```python
from build123d import *

# Parameters (mm, degrees)
SKETCH_1_W            = 179.605
SKETCH_1_H            = 31
EXTRUDE_1_DEPTH       = 8
HOLE_WIZARD_1_4_201_D = 5.1054
HOLE_WIZARD_3_8_161_D = 7.9375
FILLET_1_R            = 4


with BuildPart() as part:
    # Эскиз1 → Бобышка-Вытянуть1 (new body)
    with BuildSketch(Plane(origin=(0, 0, 0), x_dir=(1, 0, 0), z_dir=(0, 1, 0))):
        with Locations((89.8025, 15.5)):
            Rectangle(SKETCH_1_W, SKETCH_1_H)
    extrude(amount=EXTRUDE_1_DEPTH)

    # Отверстие обработанное метчиком 1/4-201 (through all)
    with Locations(Plane(origin=(0, 0, 0), x_dir=(-1, 0, 0), z_dir=(0, -1, 0))):
        with Locations((-10.475, 25), (-18.825, 25), (-27.175, 25), (-35.525, 25), (-43.875, 25), (-52.225, 25), (-60.575, 25), (-68.925, 25), (-77.275, 25), (-85.625, 25), (-93.975, 25), (-102.325, 25), (-110.675, 25), (-119.025, 25), (-127.375, 25), (-135.725, 25), (-144.075, 25), (-152.425, 25), (-160.775, 25), (-169.125, 25), (-169.125, 6), (-160.775, 6), (-152.425, 6), (-144.075, 6), (-135.725, 6), (-127.375, 6), (-119.025, 6), (-110.675, 6), (-102.325, 6), (-93.975, 6), (-85.625, 6), (-77.275, 6), (-68.925, 6), (-60.575, 6), (-52.225, 6), (-43.875, 6), (-35.525, 6), (-27.175, 6), (-18.825, 6), (-10.475, 6)):
            Hole(HOLE_WIZARD_1_4_201_D / 2)

    # Отверстие обработанное метчиком 3/8-161 (through all)
    with Locations(Plane(origin=(0, 0, 0), x_dir=(-1, 0, 0), z_dir=(0, -1, 0))):
        with Locations((-9.095, 15.5), (-20.62, 15.5), (-32.15, 15.5), (-43.68, 15.5), (-55.21, 15.5), (-66.74, 15.5), (-78.27, 15.5), (-89.8, 15.5), (-101.33, 15.5), (-112.86, 15.5), (-124.39, 15.5), (-135.92, 15.5), (-147.45, 15.5), (-158.98, 15.5), (-170.51, 15.5)):
            Hole(HOLE_WIZARD_3_8_161_D / 2)

    # Скругление1
    fillet_1_edges = [part.edges().sort_by_distance(p)[0] for p in [
        (0, 4, 0),
        (0, 4, -31),
        (179.605, 4, -31),
        (179.605, 4, 0),
    ]]
    fillet(fillet_1_edges, radius=FILLET_1_R)


solid = part.part
```
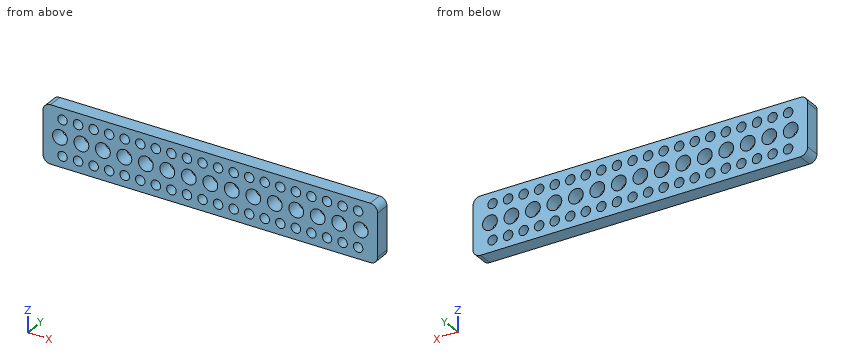
Check sheet for the modelled part. Datum: model origin and axes. Units: mm. Give positions to 0.01 mm unless a question says otherwise; leave off trailing zeros. Order: outer loops, then holes, each group sorted by start corner. A loop starts at its lowest first (then second) coordinate and runs counter-clockwise, first axis right, second up. Notation, with made-up numbers: (27, -16.5) -> (77, -16.5) arc R18 ccw to (77, 2.5) -> close; hole circle Ø4 at (-37, 13). An arc over 180 degrees is marked (long way). Use CSV: the item, a comma, the result in double quotes. Start each with the question number.
1) Sectioned sample at D-D, the plane x = 69. Record the boundary of the cut face in (y, z), plus the area to 3 significant figures.
2) Material ranges on line 1 (Z direction, x = 27.5, y = 6); line 2 (Z direction, x = 45, y = 1.5); line 3 (Z direction, x = 89.8, y = 6.5), recorded low to high. Write a range as from..to.
3) Sectioned sample at B-B, the plane z = -6. Give the number of separate pieces and of enclosed holes in the cut face, plus the area to 3 significant figures.
4) Go/stop test with a flat-tipped pin: P1, Ø8, axis at x = 77.275, z = -25, coming from the -Y side. Record where the tip stops, or that it passes through.
5) Sectioned sample at A-A, the plane x = 101.33. Record the boundary of the cut face in (y, z), plus the area to 3 significant figures.
Recorded:
1,outline,"(0, -31) -> (8, -31) -> (8, -27.55) -> (0, -27.55) -> close; (0, -22.45) -> (8, -22.45) -> (8, -18.76) -> (0, -18.76) -> close; (0, -12.24) -> (8, -12.24) -> (8, -8.55) -> (0, -8.55) -> close; (0, -3.45) -> (8, -3.45) -> (8, 0) -> (0, 0) -> close"
1,area,"114 mm2"
2,line 1,"-31..-27.53, -22.47..-8.53, -3.47..0"
2,line 2,"-31..-27.29, -22.71..-19.24, -11.76..-8.29, -3.71..0"
2,line 3,"-31..-19.47, -11.53..0"
3,separate pieces,"21"
3,enclosed holes,"0"
3,area,"620 mm2"
4,P1,"y = 0"
5,outline,"(0, -31) -> (8, -31) -> (8, -27.35) -> (0, -27.35) -> close; (0, -22.65) -> (8, -22.65) -> (8, -19.47) -> (0, -19.47) -> close; (0, -11.53) -> (8, -11.53) -> (8, -8.35) -> (0, -8.35) -> close; (0, -3.65) -> (8, -3.65) -> (8, 0) -> (0, 0) -> close"
5,area,"109 mm2"
